Could you check a few things on this drawing? It's one solid part, dimensions in mm from its lowest x, y, z. Round coordinates to 2 decimals unless told otherwise and drop trailing zeros. Order: outer loops, then holes, each group sorted by start corner. A loop starts at its lowest first (then second) coordinate and runs counter-clockwise, first axis right, second up. Notation, with made-up numbers: (-13.75, 64) -> (-4.75, 64) arc R18 cw to (-4.75, 88) -> close; hole circle Ø1 at (89, 27.25). An arc over 180 degrees is marked (long way). Use a Markdown table: item, result. Add a question column.
(1) Thinking about a two-plate mould opening in Z: for the marked faces 1, 2, 3 and 4, which applies, pulls with the +Z half, pulls with the -Z half, needs draft (parallel to the pull), parting line crosses it, or undercut?
(2) I'm going to push a flat-ended pin straight in: P1, Ø11.5, axis at y = 25.4, z = 25.4, coming from the +X side. Where does the tip first touch, or does it pass through?
(3) I want a section at C-C, the plane y = 41.5. Please give me the cut outline in (x, z) (3 decimals).
(4) If I drill on probe 1 along Y at (x, z) = (6, 25); probe 2 along X at (y, z) = (25.4, 7) (3 decimals), over which ranges is the centre line in solid material (lowest first)?
(5) I want a section at A-A, the plane z = 25.4. Please give me the cut outline in (x, y) (3 decimals), then the cut area to 3 significant figures.
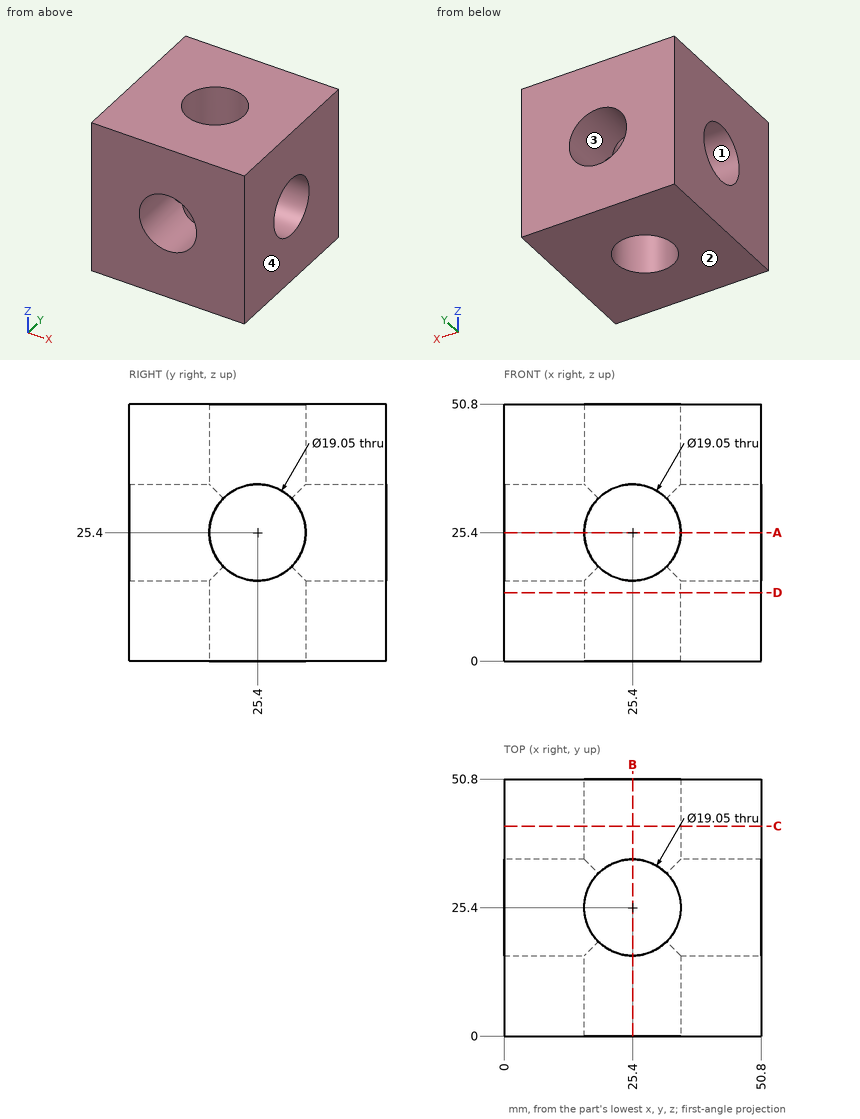
Taken from the geometry:
| question | item | result |
|---|---|---|
| 1 | face 1 | undercut |
| 1 | face 2 | pulls with the -Z half |
| 1 | face 3 | undercut |
| 1 | face 4 | needs draft |
| 2 | P1 | passes through |
| 3 | outline | (0, 0) -> (50.8, 0) -> (50.8, 50.8) -> (0, 50.8) -> close; hole circle Ø19.05 at (25.4, 25.4) |
| 4 | probe 1 | y = 0 to 15.88, 34.92 to 50.8 |
| 4 | probe 2 | x = 0 to 15.875, 34.925 to 50.8 |
| 5 | outline | (0, 0) -> (15.875, 0) -> (15.875, 15.875) -> (0, 15.875) -> close; (0, 34.925) -> (15.875, 34.925) -> (15.875, 50.8) -> (0, 50.8) -> close; (34.925, 0) -> (50.8, 0) -> (50.8, 15.875) -> (34.925, 15.875) -> close; (34.925, 34.925) -> (50.8, 34.925) -> (50.8, 50.8) -> (34.925, 50.8) -> close |
| 5 | area | 1,010 mm2 |
